```python
from build123d import *

# Parameters (mm, degrees)
SKETCH1_W               = 105
SKETCH1_H               = 4
SKETCH1_W_2             = 2
SKETCH1_H_2             = 8
BOSS_EXTRUDE1_DEPTH     = 12.5
SKETCH2_R               = 1.55
CUT_EXTRUDE2_DEPTH      = 102
CUT_EXTRUDE2_DEPTH_BACK = 5


with BuildPart() as part:
    # Sketch1 → Boss-Extrude1 (new body, symmetric)
    with BuildSketch(Plane(origin=(0, 0, 0), x_dir=(0, 0, -1), z_dir=(1, 0, 0))):
        Rectangle(SKETCH1_W, SKETCH1_H)
        Polygon((-52.5, 65), (-52.5, 2), (-48.5, 2), (-48.5, 65), (-50.5, 65), align=None)
        Polygon((48.5, 65), (48.5, 2), (52.5, 2), (52.5, 65), (50.5, 65), align=None)
        with Locations((-49.5, 69)):
            Rectangle(SKETCH1_W_2, SKETCH1_H_2)
        with Locations((49.5, 69)):
            Rectangle(SKETCH1_W_2, SKETCH1_H_2)
    extrude(amount=BOSS_EXTRUDE1_DEPTH, both=True)

    # Sketch2 → Cut-Extrude2 (cut, two sides)
    with BuildSketch(Plane(origin=(0, 0, 48.5), x_dir=(-1, 0, 0), z_dir=(0, 0, -1))) as cut_extrude2_sk:
        with Locations((-8.5, 16)):
            Circle(SKETCH2_R)
        with Locations((-8.5, 44)):
            Circle(SKETCH2_R)
        with Locations((8.5, 16)):
            Circle(SKETCH2_R)
        with Locations((8.5, 44)):
            Circle(SKETCH2_R)
    extrude(amount=CUT_EXTRUDE2_DEPTH, mode=Mode.SUBTRACT)
    extrude(cut_extrude2_sk.sketch, amount=-CUT_EXTRUDE2_DEPTH_BACK, mode=Mode.SUBTRACT)


solid = part.part
```
Work out the finished part from the listing and answer in its coordinate system (mm). A direction names the side the tool comes from. Round coordinates to 2 decimals unless told otherwise and drop trailing zeros. Write each loop counter-clockwise with the first axis right and the second up, starting at its lowest first coordinate (ties: lowest second). Pieces come first, ordered by that corner, then holes. Notation, with made-up numbers: (-23, -40) -> (1, -40) arc R27 cw to (1, -16) -> close; hole circle Ø9 at (4, -17.75). An arc over 180 degrees is marked (long way). Write each question's results on one line, items separated by ' | '.
1) The part is cut by section A-A (y = 44). Write down the section's boundary in (x, z).
Findings:
outline: (-12.5, -52.5) -> (-10.05, -52.5) -> (-10.05, -48.5) -> (-12.5, -48.5) -> close; (-12.5, 48.5) -> (-10.05, 48.5) -> (-10.05, 52.5) -> (-12.5, 52.5) -> close; (-6.95, -52.5) -> (6.95, -52.5) -> (6.95, -48.5) -> (-6.95, -48.5) -> close; (-6.95, 48.5) -> (6.95, 48.5) -> (6.95, 52.5) -> (-6.95, 52.5) -> close; (10.05, -52.5) -> (12.5, -52.5) -> (12.5, -48.5) -> (10.05, -48.5) -> close; (10.05, 48.5) -> (12.5, 48.5) -> (12.5, 52.5) -> (10.05, 52.5) -> close
2) Flat-ended cylindrical pins translate along their axes: pin 1 (3 mm diameter, centred on x = 8.5, y = 44, fed in from +Z); pin 2 (0.6 mm diameter, centred on x = -2.5, z = 51.5, fed in from +Y); pin 3 (4 mm diameter, centred on x = -3, y = 70, fed in from -Z). Find the tip coordinate at first contact, or state that the pin passes through.
Findings:
pin 1: passes through | pin 2: stops at y = 65 | pin 3: stops at z = -50.5
3) For a pull along X with two mould halves and no side action, classify faces 6 (the flat face through (-12.5, 0, -4)), 7 (the cylindrical face through (-8.298, 17.537, 50.472)), 8 (the flat face through (0, 32, 52.5)) as +X half, -X half, draft (parallel to the pull), parting line (faces both ways), or undercut.
Findings:
face 6: -X half | face 7: undercut | face 8: draft
4) Consider line 1 along X through (y, z) = (44, -50); line 2 along Y through (x, z) = (8.5, -50.45); line 3 along Y through (x, z) = (-8.5, -51). Determine where each line is inside the solid, lowest interval first. Write a range as [from, to].
Findings:
line 1: x = [-12.5, -10.05], [-6.95, 6.95], [10.05, 12.5] | line 2: y = [-2, 14.45], [17.55, 42.45], [45.55, 73] | line 3: y = [-2, 14.45], [17.55, 42.45], [45.55, 65]
5) Which of the six approach directions +Z, -Z, +X, -X, +Y, -Y give full straight-line access (tool end or side, diameter ignored) to faces 1 (the cylindrical face through (8.702, 17.537, -50.472)), 2 (the flat face through (0, 2, 1)), 3 (the flat face through (0, 69, -50.5)), 4 (the flat face through (0, 73, 50)), 5 (the flat face through (0, 69, 50.5))?
Findings:
face 1: +Z, -Z | face 2: +X, -X, +Y | face 3: -Z, +X, -X, +Y | face 4: +Z, -Z, +X, -X, +Y | face 5: +Z, +X, -X, +Y
6) The part is cut by section B-B (x = -8.5). Write down the section's boundary in (y, z), and give its area (3 significant figures).
Findings:
outline: (-2, -52.5) -> (14.45, -52.5) -> (14.45, -48.5) -> (2, -48.5) -> (2, 48.5) -> (14.45, 48.5) -> (14.45, 52.5) -> (-2, 52.5) -> close; (17.55, -52.5) -> (42.45, -52.5) -> (42.45, -48.5) -> (17.55, -48.5) -> close; (17.55, 48.5) -> (42.45, 48.5) -> (42.45, 52.5) -> (17.55, 52.5) -> close; (45.55, -52.5) -> (65, -52.5) -> (65, -50.5) -> (73, -50.5) -> (73, -48.5) -> (45.55, -48.5) -> close; (45.55, 48.5) -> (73, 48.5) -> (73, 50.5) -> (65, 50.5) -> (65, 52.5) -> (45.55, 52.5) -> close | area: 906 mm²
7) The part is cut by section C-C (y = 23). Write down the section's boundary in (x, z).
Findings:
outline: (-12.5, -52.5) -> (12.5, -52.5) -> (12.5, -48.5) -> (-12.5, -48.5) -> close; (-12.5, 48.5) -> (12.5, 48.5) -> (12.5, 52.5) -> (-12.5, 52.5) -> close
8) The part is cut by section D-D (x = -3). Write down the section's boundary in (y, z).
Findings:
outline: (-2, -52.5) -> (65, -52.5) -> (65, -50.5) -> (73, -50.5) -> (73, -48.5) -> (2, -48.5) -> (2, 48.5) -> (73, 48.5) -> (73, 50.5) -> (65, 50.5) -> (65, 52.5) -> (-2, 52.5) -> close
